Here's how the part is built. I have some questions about the finished solid (model axes, mm). Face numbers are marked on the shaded views. A direction names the side the tool comes from. Give positions to 0.01 mm unless a question says otherwise; leave off trailing zeros. Order: outer loops, then holes, each group sorted by start corner. A loop starts at its lowest first (then second) coordinate and runs counter-clockwise, first axis right, second up. Notation, with made-up numbers: M 15.5,72.5 L 70.5,72.5 A17 cw 70.5,97.5 Z; hole C 66.25,32.5 d8. An arc over 180 degrees is marked long. Use one line per item in the form item = value.
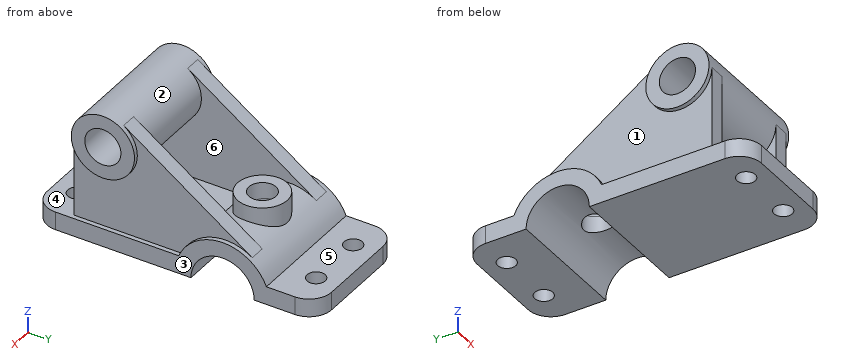
from build123d import *

# Parameters (mm, degrees)
BOSS_EXTRUDE1_DEPTH      = 28
FILLET1_R                = 10
SKETCH2_R                = 14
SKETCH2_R_2              = 8
BOSS_EXTRUDE3_DEPTH      = 28
BOSS_EXTRUDE4_START      = 7
BOSS_EXTRUDE4_DEPTH      = 7
BOSS_EXTRUDE5_REACH      = 95.814
BOSS_EXTRUDE5_END_RADIUS = 21
SKETCH5_R                = 11
SKETCH5_R_2              = 6
CUT_EXTRUDE1_DEPTH       = 94.813645093
CUT_EXTRUDE1_DEPTH_BACK  = 94.813645093
SKETCH6_R                = 6
CUT_EXTRUDE2_DEPTH       = 103.181211608
CUT_EXTRUDE2_DEPTH_BACK  = 103.181211608
SKETCH8_R                = 4
CUT_EXTRUDE3_DEPTH       = 103.181211608
CUT_EXTRUDE3_DEPTH_BACK  = 103.181211608
SKETCH9_R                = 4


with BuildPart() as part:
    # Sketch1 → Boss-Extrude1 (new, symmetric)
    with BuildSketch(Plane.YZ):
        with BuildLine():
            Line((42, 0), (14, 0))
            ThreePointArc((14, 0), (0, 14), (-14, 0))
            Line((-14, 0), (-84, 0))
            Line((-84, 0), (-84, 8))
            Line((-84, 8), (-19.416487839, 8))
            ThreePointArc((-19.416487839, 8), (0, 21), (19.416487839, 8))
            Line((19.416487839, 8), (42, 8))
            Line((42, 8), (42, 0))
        make_face()
    extrude(amount=BOSS_EXTRUDE1_DEPTH, both=True)

    # Fillet1
    fillet1_edges = [part.edges().sort_by_distance(p)[0] for p in [
        (-28, 42, 4),
        (28, -84, 4),
        (28, 42, 4),
        (-28, -84, 4),
    ]]
    fillet(fillet1_edges, radius=FILLET1_R)



with BuildPart() as body_2:
    # Sketch2 → Boss-Extrude3 (new, symmetric)
    with BuildSketch(Plane.YZ):
        with Locations(Location((-53, 45, 0), (0, 0, 270))):
            Circle(SKETCH2_R)
        with Locations(Location((-53, 45, 0), (0, 0, 270))):
            Circle(SKETCH2_R_2, mode=Mode.SUBTRACT)
    extrude(amount=BOSS_EXTRUDE3_DEPTH, both=True)


with BuildPart() as part_1:
    add(part.part)

    add(body_2.part)  # Boss-Extrude4 merges body 2
    # Sketch3 → Boss-Extrude4 (add)
    with BuildSketch(Plane.YZ.offset(19).offset(BOSS_EXTRUDE4_START)):
        with BuildLine():
            ThreePointArc((-39, 45), (-53, 31), (-67, 45))
            Line((-67, 45), (-67, 8))
            Line((-67, 8), (-19.416487839, 8))
            ThreePointArc((-19.416487839, 8), (-5.973550046, 20.132478731), (11.911075968, 17.295267251))
            Line((11.911075968, 17.295267251), (-45.059282688, 56.530178167))
            ThreePointArc((-45.059282688, 56.530178167), (-40.607057606, 51.512678314), (-39, 45))
        make_face()
    boss_extrude4 = extrude(amount=-BOSS_EXTRUDE4_DEPTH)

    # Mirror1: Boss-Extrude4 across plane
    add(boss_extrude4.mirror(Plane(origin=(0, 0, 0), x_dir=(0, 0, 1), z_dir=(1, 0, 0))))

    # Boss-Extrude5: up to this cylinder (the profile starts outside it)
    boss_extrude5_end = Plane(origin=(-10.688873, 0, 0), z_dir=(-1, 0, 0)) * Cylinder(BOSS_EXTRUDE5_END_RADIUS, 234.628, mode=Mode.PRIVATE)
    # Sketch5 → Boss-Extrude5 (add, up to the surface)
    with BuildSketch(Plane.XY.offset(28), mode=Mode.PRIVATE) as boss_extrude5_sk1:
        Circle(SKETCH5_R)
        Circle(SKETCH5_R_2, mode=Mode.SUBTRACT)
    boss_extrude5_tool1 = extrude(boss_extrude5_sk1.sketch, amount=-BOSS_EXTRUDE5_REACH, mode=Mode.PRIVATE) - boss_extrude5_end
    add(boss_extrude5_tool1.solids().sort_by_distance((-10.688873, 0, 28))[0])

    # Sketch6 → Cut-Extrude1 (cut, two sides: drawn at the far end of the back side and taken through both)
    with BuildSketch(Plane.XY.offset(28).offset(-CUT_EXTRUDE1_DEPTH_BACK)):
        Circle(SKETCH6_R)
    extrude(amount=CUT_EXTRUDE1_DEPTH + CUT_EXTRUDE1_DEPTH_BACK, mode=Mode.SUBTRACT)

    # Sketch8 → Cut-Extrude2 (cut, two sides: drawn at the far end of the back side and taken through both)
    with BuildSketch(Plane.XY.offset(8).offset(-CUT_EXTRUDE2_DEPTH_BACK)):
        with Locations((-13, 32)):
            Circle(SKETCH8_R)
        with Locations((13, 32)):
            Circle(SKETCH8_R)
    extrude(amount=CUT_EXTRUDE2_DEPTH + CUT_EXTRUDE2_DEPTH_BACK, mode=Mode.SUBTRACT)

    # Sketch9 → Cut-Extrude3 (cut, two sides: drawn at the far end of the back side and taken through both)
    with BuildSketch(Plane.XY.offset(8).offset(-CUT_EXTRUDE3_DEPTH_BACK)):
        with Locations((-13, -74)):
            Circle(SKETCH9_R)
        with Locations((13, -74)):
            Circle(SKETCH9_R)
    extrude(amount=CUT_EXTRUDE3_DEPTH + CUT_EXTRUDE3_DEPTH_BACK, mode=Mode.SUBTRACT)


solid = part_1.part
Q1. I need wall thicknesses on L1, parallel to X at y = 32, z = 3.75; L2, parallel to Y at x = -13, z = 45; L3, parallel to Y at x = 13, z = 6.25. Which ranges of each line are inside material? Lowest first, please.
Found:
L1 = -28 to -17, -9 to 9, 17 to 28
L2 = -67 to -61, -45 to -39
L3 = -84 to -78, -70 to -12.53, 12.53 to 28, 36 to 42
Q2. I'm going to push flat-ended pins straight in: pin 1 Ø2 at (x, z) = (-24, 35.5) entering from -Y; pin 2 Ø2 at (x, z) = (-2.5, 28.5) entering from +Y; pin 3 Ø6 at (x, z) = (-12, 18) entering from +Y. Where does each tip first touch, or does it pass through?
Found:
pin_1 = -67
pin_2 = 10.88
pin_3 = 14.7
Q3. I want a section at A-A on x = -13. Write out the boundary of the cut face in (y, z).
Found:
outline = M -84,0 L -78,0 L -78,8 L -84,8 Z; M -70,0 L -14,0 A14 cw 14,0 L 28,0 L 28,8 L 19.42,8 A21 ccw -19.42,8 L -70,8 Z; C -53,45 d28; M 36,0 L 42,0 L 42,8 L 36,8 Z; hole C -53,45 d16
Q4. I want a section at C-C on x = 0. Write out the boundary of the cut face in (y, z), then the cut area to 3 significant figures.
Found:
outline = M -84,0 L -14,0 A14 cw -6,12.65 L -6,28 L -11,28 L -11,17.89 A21 ccw -19.42,8 L -84,8 Z; C -53,45 d28; M 6,12.65 A14 cw 14,0 L 42,0 L 42,8 L 19.42,8 A21 ccw 11,17.89 L 11,28 L 6,28 Z; hole C -53,45 d16
area = 1,480 mm²
Q5. I want a section at D-D on z = 26. Write out the boundary of the cut face in (x, y).
Found:
outline = M -26,-67 L -19,-67 L -19,-0.73 L -26,-0.73 Z; C 0,0 d22; M 19,-67 L 26,-67 L 26,-0.73 L 19,-0.73 Z; hole C 0,0 d12
Q6. On a 3-axis mill with a long thin cutter (end or side, diameter ignored), from which of +Z, -Z, +X, -X, +Y, -Y can I reach the whole of each face in a straight line? I mean the marked faces 4, 5 and 6. Say none if no direction works.
Found:
face_4 = -Y
face_5 = +Z, +X, -X, +Y
face_6 = none
Q7. I want a section at B-B on y = -53. Write out the boundary of the cut face in (x, z), then the cut area to 3 significant figures.
Found:
outline = M -28,0 L 28,0 L 28,8 L 26,8 L 26,31 L 28,31 L 28,37 L -28,37 L -28,31 L -26,31 L -26,8 L -28,8 Z; M -28,53 L 28,53 L 28,59 L -28,59 Z; hole M -19,8 L 19,8 L 19,31 L -19,31 Z
area = 1,440 mm²
Q8. Thinking about a two-plate mould opening in X: for the marked faces 1, 2 and 3, which applies, +X half, -X half, draft (parallel to the pull), parting line (faces both ways), or undercut?
Found:
face_1 = -X half
face_2 = undercut
face_3 = +X half
